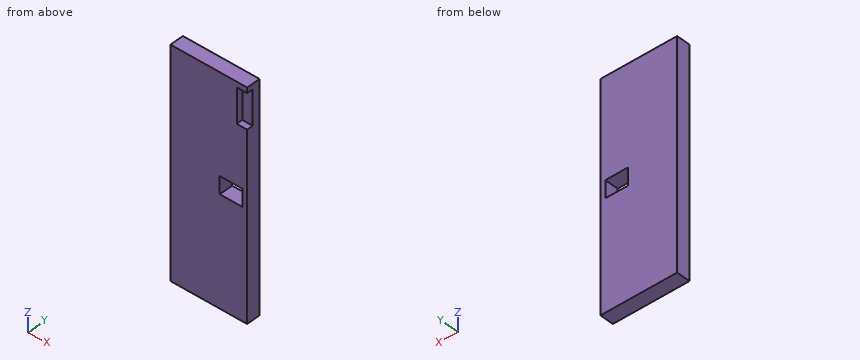
from build123d import *

# Parameters (mm, degrees)
SKETCH1_W           = 100
SKETCH1_H           = 292
BOSS_EXTRUDE1_DEPTH = 9
SKETCH2_W           = 29.4
SKETCH2_H           = 22.4
CUT_EXTRUDE1_DEPTH  = 19
SKETCH3_W           = 13.5
SKETCH3_H           = 45
CUT_EXTRUDE2_DEPTH  = 8


with BuildPart() as part:
    # Sketch1 → Boss-Extrude1 (new body, symmetric)
    with BuildSketch(Plane(origin=(0, 0, 0), x_dir=(1, 0, 0), z_dir=(0, 1, 0))):
        Rectangle(SKETCH1_W, SKETCH1_H)
    extrude(amount=BOSS_EXTRUDE1_DEPTH, both=True)

    # Sketch2 → Cut-Extrude1 (cut, through all)
    with BuildSketch(Plane.XZ.offset(9)):
        with Locations((29, 6.5)):
            Rectangle(SKETCH2_W, SKETCH2_H)
    extrude(amount=-CUT_EXTRUDE1_DEPTH, mode=Mode.SUBTRACT)

    # Sketch3 → Cut-Extrude2 (cut)
    with BuildSketch(Plane.XZ.offset(9)):
        with Locations((43.25, 116.521105827)):
            Rectangle(SKETCH3_W, SKETCH3_H)
    extrude(amount=-CUT_EXTRUDE2_DEPTH, mode=Mode.SUBTRACT)


solid = part.part
Geometry check sheet. Reference: the model listing, model coordinates, mm. Give positions to 0.01 mm unless a question says otherwise; leave off trailing zeros. Order: outer loops, then holes, each group sorted by start corner. A loop starts at its lowest first (then second) coordinate and runs counter-clockwise, first axis right, second up.
1) Material ranges on probe 1 along Z at (x, y) = (36, -1.25); probe 2 along Z at (x, y) = (44.5, -6.75); probe 3 along X at (y, z) = (-6.5, 109.5), recorded low to high.
Results are:
probe 1: z = -146 to -4.7, 17.7 to 146
probe 2: z = -146 to 94.02, 139.02 to 146
probe 3: x = -50 to 36.5
2) Cross-section at C-C (z = 112). Record the boundary of the cut face in (x, y), then the cut area to 3 significant figures.
Results are:
outline: (-50, -9) - (36.5, -9) - (36.5, -1) - (50, -1) - (50, 9) - (-50, 9) - close
area: 1,690 mm2
3) Cross-section at B-B (x = 34). Record the boundary of the cut face in (y, z), then the cut area to 3 significant figures.
Results are:
outline: (-9, -146) - (9, -146) - (9, -4.7) - (-9, -4.7) - close; (-9, 17.7) - (9, 17.7) - (9, 146) - (-9, 146) - close
area: 4,850 mm2
4) Cross-section at A-A (z = 13). Record the boundary of the cut face in (x, y), then the cut area to 3 significant figures.
Results are:
outline: (-50, -9) - (14.3, -9) - (14.3, 9) - (-50, 9) - close; (43.7, -9) - (50, -9) - (50, 9) - (43.7, 9) - close
area: 1,270 mm2
5) Gauge pin test, flat ends, axial feed: pin 1 (4 mm diameter, centred on x = 42.5, z = 110.5, fed in from -Y); pin 2 (6.5 mm diameter, centred on y = -5.5, z = 126, fed in from +X). Record the tip position at first contact, or that the pin passes through.
Results are:
pin 1: stops at y = -1
pin 2: stops at x = 36.5
